from build123d import *

# Parameters (mm, degrees)
BOSS_EXTRUDE1_DEPTH = 2
SKETCH3_W           = 13
SKETCH3_H           = 20
CUT_EXTRUDE1_DEPTH  = 11.5
SKETCH4_R           = 0.75
CUT_EXTRUDE2_DEPTH  = 4.5
SKETCH5_R           = 5
CUT_EXTRUDE3_DEPTH  = 10


with BuildPart() as part:
    # Sketch2 → Boss-Extrude1 (new body)
    with BuildSketch(Plane.XY):
        with BuildLine():
            Line((-7.651598568, -15.738584414), (-7.651598568, -21.41907999))
            Line((-7.651598568, -21.41907999), (-22.651598568, -21.41907999))
            Line((-22.651598568, -21.41907999), (-22.651598568, -86.41907999))
            Line((-22.651598568, -86.41907999), (22.348401432, -86.41907999))
            Line((22.348401432, -86.41907999), (22.348401432, -21.41907999))
            Line((22.348401432, -21.41907999), (7.348401432, -21.41907999))
            Line((7.348401432, -21.41907999), (7.348401432, -15.882411542))
            ThreePointArc((7.348401432, -15.882411542), (0.167790603, 17.49919559), (-7.651598568, -15.738584414))
        make_face()
    extrude(amount=BOSS_EXTRUDE1_DEPTH)

    # Sketch3 → Cut-Extrude1 (cut)
    with BuildSketch(Plane.XY.offset(2)):
        with Locations((9.306683573, -64.699747406)):
            Rectangle(SKETCH3_W, SKETCH3_H)
        with Locations((-5.874609334, -39.631347468)):
            Rectangle(SKETCH3_W, SKETCH3_H)
    extrude(amount=-CUT_EXTRUDE1_DEPTH, mode=Mode.SUBTRACT)

    # Sketch4 → Cut-Extrude2 (cut)
    with BuildSketch(Plane.XY.offset(2)):
        with Locations((-5.874609334, -27.679486822)):
            Circle(SKETCH4_R)
        with Locations((-5.874609334, -55.313369489)):
            Circle(SKETCH4_R)
        with Locations((9.318214062, -52.431887672)):
            Circle(SKETCH4_R)
        with Locations((9.290500092, -80.290661027)):
            Circle(SKETCH4_R)
    extrude(amount=-CUT_EXTRUDE2_DEPTH, mode=Mode.SUBTRACT)

    # Sketch5 → Cut-Extrude3 (cut)
    with BuildSketch(Plane.XY.offset(2)):
        with Locations((-12.686703833, -77.415205598)):
            Circle(SKETCH5_R)
    extrude(amount=-CUT_EXTRUDE3_DEPTH, mode=Mode.SUBTRACT)


solid = part.part
Here's how the part is built. I have some questions about the finished solid (model axes, mm). A direction names the side the tool comes from. Round coordinates to 2 decimals unless told otherwise and drop trailing zeros. Loops run counter-clockwise (first coordinate to the right, second up) from the corner with the lowest first, then second, coordinate; pieces in that order, holes last.
1. If we section it at B-B on x = -16.5: Write out the boundary of the cut face in (y, z), plus the area to 3 significant figures.
Answer list:
outline: (-86.42, 0) - (-80.65, 0) - (-80.65, 2) - (-86.42, 2) - close; (-74.18, 0) - (-21.42, 0) - (-21.42, 2) - (-74.18, 2) - close; (-5.83, 0) - (5.83, 0) - (5.83, 2) - (-5.83, 2) - close
area: 140 mm2
2. Which directions (+Z, -Z, +X, -X, +Y, -Y) give clear straight access to the entire face, cutting with the end or side of a thin tool? Please do faces 1 (the face through (15, -21.419, 1)), 2 (the face through (2.807, -65, 1)), 3 (the face through (-15, -21.419, 1)).
Answer list:
face 1: +Z, -Z, +X
face 2: +Z, -Z
face 3: +Z, -Z, -X
3. If we section it at D-D on y = 0: Write out the boundary of the cut face in (x, z), plus the area to 3 significant figures.
Answer list:
outline: (-17.5, 0) - (17.5, 0) - (17.5, 2) - (-17.5, 2) - close
area: 70.0 mm2
4. If we section it at C-C on z = 1.6: Write out the boundary of the cut face in (x, y).
Answer list:
outline: (-22.65, -86.42) - (22.35, -86.42) - (22.35, -21.42) - (7.35, -21.42) - (7.35, -15.88) arc R17.5 ccw (long way) to (-7.65, -15.74) - (-7.65, -21.42) - (-22.65, -21.42) - close; hole circle Ø10 at (-12.69, -77.42); hole (-12.37, -49.63) - (0.63, -49.63) - (0.63, -29.63) - (-12.37, -29.63) - close; hole circle Ø1.5 at (-5.87, -55.31); hole circle Ø1.5 at (-5.87, -27.68); hole (2.81, -74.7) - (15.81, -74.7) - (15.81, -54.7) - (2.81, -54.7) - close; hole circle Ø1.5 at (9.29, -80.29); hole circle Ø1.5 at (9.32, -52.43)
5. If we section it at A-A on y = -39: Write out the boundary of the cut face in (x, z).
Answer list:
outline: (-22.65, 0) - (-12.37, 0) - (-12.37, 2) - (-22.65, 2) - close; (0.63, 0) - (22.35, 0) - (22.35, 2) - (0.63, 2) - close
6. If I drill on line 1 along X through (y, z) = (-74.5, 0.4); line 2 along Y through (x, z) = (-16, 1.9); line 3 along Y through (x, z) = (15, 0.95), over which ranges is the centre line in solid material (lowest first)?
Answer list:
line 1: x = -22.65 to -16.75, -8.62 to 2.81, 15.81 to 22.35
line 2: y = -86.42 to -81.16, -73.67 to -21.42, -7.09 to 7.09
line 3: y = -86.42 to -74.7, -54.7 to -21.42, -9.01 to 9.01
7. For P1, Ø1, axis at x = -4.5, z = 0, coming from the +Y side; P2, Ø1, axis at x = 10.5, z = 1, coming from the +Y side; P3, Ø1.7, axis at x = 9.29, y = -80.29, coming from the -Z side; P4, Ø1, axis at x = 11, z = 1, coming from the +Y side, each with a flat end and sliding along its axis, tell me the tip position at first contact or that it passes through.
Answer list:
P1: stops at y = 17.04
P2: stops at y = 14.36
P3: stops at z = 0
P4: stops at y = 14
8. We'd pull the mould along X, two halves only. Please class faces 4 (the face through (0, -86.419, 1)), 5 (the face through (-13.771, -82.296, 1.014)), 6 (the face through (22.348, -54, 1)): +X half, -X half, draft (parallel to the pull), parting line (faces both ways), or undercut.
Answer list:
face 4: draft
face 5: undercut
face 6: +X half
